Work out the finished part from the listing and answer in its coordinate system (mm). A direction names the side the tool comes from. Round coordinates to 2 decimals unless told otherwise and drop trailing zeros. Loops run counter-clockwise (first coordinate to the right, second up) from the corner with the lowest first, then second, coordinate; pieces in that order, holes last. Notation, with made-up numbers: (80.25, 43) -> (84.25, 43) arc R14 cw to (84.25, 64) -> close; hole circle Ø11 at (-9.5, 88). An arc over 180 degrees is marked (long way). Use one line per item in the form item = value.
```python
from build123d import *

# Parameters (mm, degrees)
SKETCH1_W           = 309.5625
SKETCH1_H           = 231.775
SKETCH1_W_2         = 265.1125
SKETCH1_H_2         = 187.325
SKETCH1_W_3         = 227.0125
SKETCH1_H_3         = 150.8125
BOSS_EXTRUDE1_DEPTH = 9.525
SKETCH1_3_W         = 265.1125
SKETCH1_3_H         = 187.325
SKETCH1_3_W_2       = 227.0125
SKETCH1_3_H_2       = 150.8125
BOSS_EXTRUDE2_DEPTH = 9.525
FILLET1_R           = 12.7
CUT_EXTRUDE1_START  = 9.525
SKETCH1_4_W         = 265.1125
SKETCH1_4_H         = 187.325
SKETCH1_4_W_2       = 227.0125
SKETCH1_4_H_2       = 150.8125
CUT_EXTRUDE1_DEPTH  = 6.35
FILLET2_R           = 6.35
FILLET3_R           = 12.7
FILLET4_R           = 9.525


with BuildPart() as part:
    # Sketch1 → Boss-Extrude1 (new body)
    # profile 1 of 2: a face of its own
    with BuildSketch(Plane.XY):
        Rectangle(SKETCH1_W, SKETCH1_H)
        Rectangle(SKETCH1_W_2, SKETCH1_H_2, mode=Mode.SUBTRACT)
    # profile 2 of 2: a face of its own
    with BuildSketch(Plane.XY):
        Rectangle(SKETCH1_W_2, SKETCH1_H_2)
        Rectangle(SKETCH1_W_3, SKETCH1_H_3, mode=Mode.SUBTRACT)
    extrude(amount=BOSS_EXTRUDE1_DEPTH)

    # Sketch1<3> → Boss-Extrude2 (add)
    with BuildSketch(Plane.XY):
        Rectangle(SKETCH1_3_W, SKETCH1_3_H)
        Rectangle(SKETCH1_3_W_2, SKETCH1_3_H_2, mode=Mode.SUBTRACT)
    extrude(amount=-BOSS_EXTRUDE2_DEPTH)

    # Fillet1
    fillet1_edges = [part.edges().sort_by_distance(p)[0] for p in [
        (-154.78125, -115.8875, 4.7625),
        (-154.78125, 115.8875, 4.7625),
        (154.78125, 115.8875, 4.7625),
        (154.78125, -115.8875, 4.7625),
        (132.55625, -93.6625, -4.7625),
        (-132.55625, -93.6625, -4.7625),
        (-132.55625, 93.6625, -4.7625),
        (132.55625, 93.6625, -4.7625),
    ]]
    fillet(fillet1_edges, radius=FILLET1_R)

    # Sketch1<4> → Cut-Extrude1 (cut)
    with BuildSketch(Plane.XY.offset(CUT_EXTRUDE1_START)):
        Rectangle(SKETCH1_4_W, SKETCH1_4_H)
        Rectangle(SKETCH1_4_W_2, SKETCH1_4_H_2, mode=Mode.SUBTRACT)
    extrude(amount=-CUT_EXTRUDE1_DEPTH, mode=Mode.SUBTRACT)

    # Fillet2
    fillet2_edges = [part.edges().sort_by_distance(p)[0] for p in [
        (-113.50625, 75.40625, -3.175),
        (113.50625, 75.40625, -3.175),
        (-113.50625, -75.40625, -3.175),
        (113.50625, -75.40625, -3.175),
    ]]
    fillet(fillet2_edges, radius=FILLET2_R)

    # Fillet3
    fillet3_edges = [part.edges().sort_by_distance(p)[0] for p in [
        (-132.55625, -93.6625, 6.35),
        (-132.55625, 93.6625, 6.35),
        (132.55625, 93.6625, 6.35),
        (132.55625, -93.6625, 6.35),
    ]]
    fillet(fillet3_edges, radius=FILLET3_R)

    # Fillet4
    fillet4_edges = [part.edges().sort_by_distance(p)[0] for p in [
        (-151.061506121, -112.167756121, 9.525),
        (0, -115.8875, 9.525),
        (151.061506121, -112.167756121, 9.525),
        (154.78125, 0, 9.525),
        (151.061506121, 112.167756121, 9.525),
        (0, 115.8875, 9.525),
        (-151.061506121, 112.167756121, 9.525),
        (-154.78125, 0, 9.525),
    ]]
    fillet(fillet4_edges, radius=FILLET4_R - 0.0001)  # a hair under: the kernel refuses the full size


solid = part.part
```
(1) Consider L1, parallel to Y at x = 45, z = -5; L2, parallel to X at y = -30.5, z = -2; L3, parallel to X at y = -70, z = -5. Determine where each line is inside the solid, lowest interval first.
Completed:
L1 = -93.66 to -75.41, 75.41 to 93.66
L2 = -132.56 to -113.51, 113.51 to 132.56
L3 = -132.56 to -113.44, 113.44 to 132.56
(2) For faces 1 (the cylindrical face through (128.935, -89.843, -4.829)), 2 (the flat face through (-2, 93.662, 6)), 3 (the flat face through (113.506, -1, -3)), 4 (the cylindrical face through (-128.935, -89.843, -4.829)), 5 (the flat face through (-2, -101, 0)), determine the directions among +Z, -Z, +X, -X, +Y, -Y from which every point of the face is accessible in a straight line to the end or side of a thin tool.
Completed:
face_1 = -Z, +X, -Y
face_2 = +Z
face_3 = +Z, -Z
face_4 = -Z, -X, -Y
face_5 = -Z
(3) Given P1, Ø10, axis at x = -39, z = -6, coming from the +Y side; P2, Ø3, axis at y = 9, z = 5.5, coming from the -X side; P3, Ø3, axis at y = -17, z = 5.5, coming from the +X side, each flat-ended and moving along its own axis, determine where each tip first touches the part or whether it passes through.
Completed:
P1 = 93.66
P2 = -153.9
P3 = 153.9
(4) Find section C-C, the plane z = -6. Write down the section's boundary in (x, y).
Completed:
outline = (-132.56, -80.96) arc R12.7 ccw to (-119.86, -93.66) -> (119.86, -93.66) arc R12.7 ccw to (132.56, -80.96) -> (132.56, 80.96) arc R12.7 ccw to (119.86, 93.66) -> (-119.86, 93.66) arc R12.7 ccw to (-132.56, 80.96) -> close; hole (-113.51, -69.06) arc R6.35 ccw to (-107.16, -75.41) -> (107.16, -75.41) arc R6.35 ccw to (113.51, -69.06) -> (113.51, 69.06) arc R6.35 ccw to (107.16, 75.41) -> (-107.16, 75.41) arc R6.35 ccw to (-113.51, 69.06) -> close
(5) For a pull along Y with two mould halves and no side action, classify faces 6 (the flat face through (-2, -82, -9.525)), 7 (the cylindrical face through (1.99, 113.02, 6.81)), 8 (the cylindrical face through (-111.597, 73.595, -3.264)) as +Y half, -Y half, draft (parallel to the pull), parting line (faces both ways), or undercut.
Completed:
face_6 = draft
face_7 = +Y half
face_8 = undercut
